Model file for the job. Use its own axes, mm. Face numbers are marked on the shaded views. A direction names the side the tool comes from. Give positions to 0.01 mm unless a question says otherwise; leave off trailing zeros. Order: outer loops, then holes, each group sorted by start corner. A loop starts at its lowest first (then second) coordinate and runs counter-clockwise, first axis right, second up. Notation, with made-up numbers: (30, 3.25) -> (45, 3.25) arc R5 cw to (45, 7.25) -> close; hole circle Ø6 at (39.25, 17). An arc over 180 degrees is marked (long way). Use CSV: the item, a comma, the result in double quotes. Start each with the question number.
1. Drop flat-ended pins along their axis: pin 1 (10 mm diameter, centred on y = 2.5, z = -17, fed in from +X); pin 2 (4.5 mm diameter, centred on y = 15.81, z = -19.05, fed in from -X); pin 3 (12 mm diameter, centred on x = 86.5, z = -31, fed in from +Y); pin 4 (1.5 mm diameter, centred on y = 10.5, z = -29.5, fed in from -X). Give the stop position or say it passes through.
2. Cut at A-A on x = 76.2. List the corners of the cut face in (y, z), then the cut area to 3 significant figures.
3. Cut at D-D on z = -3. List the corners of the cut face in (x, y) (1 decimal).
4. 3-axis set-ups, long thin cutter, end or side, ignore diameter. For the marked faces 1 and 2: which of +Z, -Z, +X, -X, +Y, -Y reach the whole face in a straight line?
5. Cut at B-B on y = 14.75. List the corners of the cut face in (x, z), then the cut area to 3 significant figures.
6. Wall check: line 1 (Y direction, x = 47, z = -20); line 2 (X direction, y = 18.75, z = -27.5); line 3 (Y direction, x = 17.1, z = -6.35). Give the ranges that are in metal, low to high. Write a range as from..to.
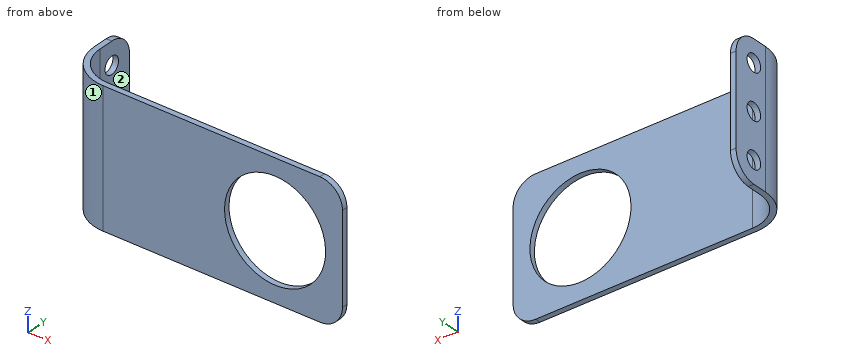
```python
from build123d import *

# Parameters (mm, degrees)
SKETCH1_W                  = 19.05
SKETCH1_H                  = 38.1
SKETCH1_R                  = 2.425
SKETCH1_R_2                = 14.2875
BOSS_EXTRUDE2_DEPTH        = 1.5875
FILLET2_R                  = 6.35
SKETCHED_BEND2_OUTLINE_W   = 1.5875
SKETCHED_BEND2_OUTLINE_H   = 38.1
SKETCHED_BEND2_DEPTH       = 17.527391426
SKETCHED_START             = 15.939891426
SKETCHED_BEND2_2_OUTLINE_R = 2.425
SKETCHED_BEND2_2_DEPTH     = 11.5875
SKETCHED_START_2           = -38.1
SKETCHED_BEND2_3_DEPTH     = 38.1


with BuildPart() as part:
    # Sketch1 → Boss-Extrude2 (new body)
    # profile 1 of 3: a face of its own
    with BuildSketch(Plane(origin=(0, 0, 0), x_dir=(1, 0, 0), z_dir=(0, 1, 0))):
        with Locations((9.525, 19.05)):
            Rectangle(SKETCH1_W, SKETCH1_H)
        with Locations(Location((6.35, 6.35, 0), (0, 0, 270))):
            Circle(SKETCH1_R, mode=Mode.SUBTRACT)
        with Locations(Location((6.35, 19.05, 0), (0, 0, 270))):
            Circle(SKETCH1_R, mode=Mode.SUBTRACT)
        with Locations(Location((6.35, 31.75, 0), (0, 0, 270))):
            Circle(SKETCH1_R, mode=Mode.SUBTRACT)
    # profile 2 of 3: a face of its own
    with BuildSketch(Plane(origin=(0, 0, 0), x_dir=(1, 0, 0), z_dir=(0, 1, 0))):
        Polygon((19.05, 38.1), (19.05, 0), (50.8, 0), (95.25, 0), (95.25, 38.1), (50.8, 38.1), align=None)
        with Locations(Location((76.2, 19.05, 0), (0, 0, 270))):
            Circle(SKETCH1_R_2, mode=Mode.SUBTRACT)
    # profile 3 of 3: a face of its own
    with BuildSketch(Plane(origin=(0, 0, 0), x_dir=(1, 0, 0), z_dir=(0, 1, 0))):
        Polygon((19.05, 38.1), (19.05, 0), (50.8, 0), (95.25, 0), (95.25, 38.1), (50.8, 38.1), align=None)
        with Locations(Location((76.2, 19.05, 0), (0, 0, 270))):
            Circle(SKETCH1_R_2, mode=Mode.SUBTRACT)
    extrude(amount=BOSS_EXTRUDE2_DEPTH)

    # Fillet2
    fillet2_edges = [part.edges().sort_by_distance(p)[0] for p in [
        (0, 0.79375, 0),
        (0, 0.79375, -38.1),
        (95.25, 0.79375, -38.1),
        (95.25, 0.79375, 0),
    ]]
    fillet(fillet2_edges, radius=FILLET2_R)

    # Sketched Bend2: read off the stored shape, not the designer's step
    # Sketched Bend2 outline → Sketched Bend2 (cut)
    with BuildSketch(Plane.YZ):
        with Locations((0.79375, -19.05)):
            Rectangle(SKETCHED_BEND2_OUTLINE_W, SKETCHED_BEND2_OUTLINE_H)
    extrude(amount=SKETCHED_BEND2_DEPTH, mode=Mode.SUBTRACT)

    # Sketched Bend2 2 outline → Sketched Bend2 2 (add)
    with BuildSketch(Plane.YZ.offset(SKETCHED_START)):
        with BuildLine():
            Line((1.5875, -38.1), (15.810108574, -38.1))
            ThreePointArc((15.810108574, -38.1), (20.300236634, -36.240128061), (22.160108574, -31.75))
            Line((22.160108574, -31.75), (22.160108574, -6.35))
            ThreePointArc((22.160108574, -6.35), (20.300236634, -1.859871939), (15.810108574, 0))
            Line((15.810108574, 0), (1.5875, 0))
            Line((1.5875, 0), (1.5875, -38.1))
        make_face()
        with Locations((15.810108574, -31.75)):
            Circle(SKETCHED_BEND2_2_OUTLINE_R, mode=Mode.SUBTRACT)
        with Locations((15.810108574, -19.05)):
            Circle(SKETCHED_BEND2_2_OUTLINE_R, mode=Mode.SUBTRACT)
        with Locations((15.810108574, -6.35)):
            Circle(SKETCHED_BEND2_2_OUTLINE_R, mode=Mode.SUBTRACT)
    extrude(amount=SKETCHED_BEND2_2_DEPTH)

    # Sketched Bend2 3 outline → Sketched Bend2 3 (cut)
    with BuildSketch(Plane.XY.offset(SKETCHED_START_2)):
        with BuildLine():
            ThreePointArc((27.527391426, 0), (19.333791599, 3.393900173), (15.939891426, 11.5875))
            Line((15.939891426, 11.5875), (15.939891426, 1.5875))
            Line((15.939891426, 1.5875), (17.527391426, 1.5875))
            Line((17.527391426, 1.5875), (17.527391426, 0))
            Line((17.527391426, 0), (27.527391426, 0))
        make_face()
        with BuildLine():
            Line((17.527391426, 22.160108574), (17.527391426, 11.5875))
            ThreePointArc((17.527391426, 11.5875), (20.456323614, 4.516432188), (27.527391426, 1.5875))
            Line((27.527391426, 1.5875), (27.527391426, 22.160108574))
            Line((27.527391426, 22.160108574), (17.527391426, 22.160108574))
        make_face()
    extrude(amount=SKETCHED_BEND2_3_DEPTH, mode=Mode.SUBTRACT)


solid = part.part
```
Verdict:
1,pin 1,"x = 95.25"
1,pin 2,"through"
1,pin 3,"y = 1.59"
1,pin 4,"x = 15.94"
2,outline,"(0, -38.1) -> (1.59, -38.1) -> (1.59, -33.34) -> (0, -33.34) -> close; (0, -4.76) -> (1.59, -4.76) -> (1.59, 0) -> (0, 0) -> close"
2,area,"15.1 mm^2"
3,outline,"(15.9, 11.6) arc R11.6 ccw to (27.5, 0) -> (94.3, 0) -> (94.3, 1.6) -> (27.5, 1.6) arc R10 cw to (17.5, 11.6) -> (17.5, 21.2) -> (15.9, 21.2) -> close"
4,face 1,"+Z, -Z, -X, -Y"
4,face 2,"+Z, -Z, +X, +Y"
5,outline,"(15.94, -38.1) -> (17.53, -38.1) -> (17.53, -33.93) -> (15.94, -33.93) -> close; (15.94, -29.57) -> (17.53, -29.57) -> (17.53, -21.23) -> (15.94, -21.23) -> close; (15.94, -16.87) -> (17.53, -16.87) -> (17.53, -8.53) -> (15.94, -8.53) -> close; (15.94, -4.17) -> (17.53, -4.17) -> (17.53, 0) -> (15.94, 0) -> close"
5,area,"39.7 mm^2"
6,line 1,"0..1.59"
6,line 2,"15.94..17.53"
6,line 3,"6.53..13.39, 18.24..22.16"
